Build history of the part. All positions in model axes, mm. A direction names the side the tool comes from. Round coordinates to 2 decimals unless told otherwise and drop trailing zeros. Order: outer loops, then holes, each group sorted by start corner. A loop starts at its lowest first (then second) coordinate and runs counter-clockwise, first axis right, second up. Notation, with made-up numbers: M 83,-32 L 103,-32 A22 ccw 103,-21 Z; hole C -11,17.25 d8. An arc over 180 degrees is marked long. One line per item, written item: value. Start each with the question number.
Item 1: Two-plate mould, pull along Z, no slides. Class faces 4 (the flat face through (15, 86, -42.61)), 5 (the flat face through (25, 69, -62.61)), 6 (the flat face through (162.537, 69, 8)): +Z half, -Z half, draft (parallel to the pull), parting line (faces both ways), or undercut.
Item 2: Band-saw the part on A-A, the plane x = 82.5. Write the cut outline in (y, z).
Item 3: Band-saw the part on B-B, the plane y = 132. Write the cut outline in (x, z), then the cut area to 3 significant figures.
Item 4: Probe L1, parallel to Z at x = 61, y = 136; L2, parallel to Y at x = -86, z = -30.5; L3, parallel to Z at x = 123.5, y = 128. List the from-to ranges inside material, lowest first.
Item 5: Pin check, flat tips, straight feed: pin 1 (5 mm diameter, centred on x = -89.46, z = 7.39, fed in from -Y); pin 2 (1 mm diameter, centred on x = 134.5, y = 97.5, fed in from +Z); pin 3 (6.5 mm diameter, centred on y = 11.5, z = 18.5, fed in from -X); pin 4 (4 mm diameter, centred on x = 108, z = 78, fed in from +Y). Stop position of each tip, or through.
Item 6: Band-saw the part on D-D, the plane y = 113. Write the cut outline in (x, z).
Item 7: Tool access for faces 1 (the flat face through (142.537, 86, 8)), 2 (the flat face through (115.537, 135, 93)), 3 (the flat face through (-60, 20, 7)): list every direction of +Z, -Z, +X, -X, +Y, -Y with a clear straight run to the whole face (end or side of a thin tool).
Item 8: Band-saw the part on C-C, the plane z = -32.5. Write the cut outline in (x, y).
```python
from build123d import *

# Parameters (mm, degrees)
SKETCH_1_W          = 272
SKETCH_1_H          = 140
EXTRUDE_1_DEPTH     = 140
SKETCH_2_W          = 252
SKETCH_2_H          = 100
CUT_EXTRUDE_1_DEPTH = 110
SKETCH_3_W          = 100
SKETCH_3_H          = 13
CUT_EXTRUDE_2_DEPTH = 100
SKETCH_7_R          = 3
CUT_EXTRUDE_3_DEPTH = 211.967749748
SKETCH_8_W          = 12
SKETCH_8_H          = 12
EXTRUDE_2_DEPTH     = 10
SKETCH_9_R          = 14.49
SKETCH_9_R_2        = 4.49
EXTRUDE_1_2_DEPTH   = 12
SKETCH_11_R         = 4.49
CUT_EXTRUDE_5_DEPTH = 298.354040116


with BuildPart() as part:
    # 草圖1 → Extrude 1 (new body)
    with BuildSketch(Plane(origin=(0, 0, 0), x_dir=(1, 0, 0), z_dir=(0, 1, 0))):
        with Locations((26.536585366, -7.390243902)):
            Rectangle(SKETCH_1_W, SKETCH_1_H)
    extrude(amount=EXTRUDE_1_DEPTH)

    # 草圖2 → 除料-伸長1 (cut)
    with BuildSketch(Plane(origin=(0, 140, 0), x_dir=(1, 0, 0), z_dir=(0, 1, 0))):
        with Locations((16.536585366, -7.390243902)):
            Rectangle(SKETCH_2_W, SKETCH_2_H)
    extrude(amount=-CUT_EXTRUDE_1_DEPTH, mode=Mode.SUBTRACT)

    # 草圖3 → 除料-伸長2 (cut)
    with BuildSketch(Plane.ZY.offset(109.463414634)):
        with Locations((7.390243902, 13.5)):
            Rectangle(SKETCH_3_W, SKETCH_3_H)
    extrude(amount=-CUT_EXTRUDE_2_DEPTH, mode=Mode.SUBTRACT)

    # 草圖7 → 除料-伸長3 (cut, through all)
    with BuildSketch(Plane(origin=(0, 30, 0), x_dir=(1, 0, 0), z_dir=(0, 1, 0))):
        with Locations(Location((-89.463414634, -7.390243902, 0), (0, 0, 270))):
            Circle(SKETCH_7_R)
    extrude(amount=-CUT_EXTRUDE_3_DEPTH, mode=Mode.SUBTRACT)

    # 草圖8 → 填料-伸長2 (add)
    with BuildSketch(Plane.XY.offset(77.390243902)):
        with Locations((121.536585366, 126)):
            Rectangle(SKETCH_8_W, SKETCH_8_H)
    extrude(amount=EXTRUDE_2_DEPTH)

    # 草圖9 → Extrude 1 2 (add)
    with BuildSketch(Plane(origin=(127.536585366, 0, 0), x_dir=(0, 0, -1), z_dir=(1, 0, 0))):
        with Locations((-89.390243902, 132)):
            Circle(SKETCH_9_R)
        with Locations((-89.390243902, 132)):
            Circle(SKETCH_9_R_2, mode=Mode.SUBTRACT)
    extrude(amount=-EXTRUDE_1_2_DEPTH)

    # 草圖11 → 除料-伸長5 (cut, through all)
    with BuildSketch(Plane(origin=(127.536585366, 0, 0), x_dir=(0, 0, -1), z_dir=(1, 0, 0))):
        with Locations((-89.390243902, 132)):
            Circle(SKETCH_11_R)
    extrude(amount=-CUT_EXTRUDE_5_DEPTH, mode=Mode.SUBTRACT)


solid = part.part
```
Output:
1. face 4: undercut
1. face 5: -Z half
1. face 6: draft
2. outline: M 0,-62.61 L 140,-62.61 L 140,-42.61 L 30,-42.61 L 30,57.39 L 140,57.39 L 140,77.39 L 0,77.39 Z
3. outline: M -109.46,-62.61 L 162.54,-62.61 L 162.54,77.39 L 127.54,77.39 L 127.54,84.9 L 115.54,84.9 L 115.54,77.39 L -109.46,77.39 L -109.46,57.39 L 142.54,57.39 L 142.54,-42.61 L -109.46,-42.61 Z; M 115.54,93.88 L 127.54,93.88 L 127.54,103.88 L 115.54,103.88 Z
3. area: 13,100 mm²
4. L1: z = -62.61 to -42.61, 57.39 to 77.39
4. L2: y = 0 to 7, 20 to 30
4. L3: z = -62.61 to -42.61, 57.39 to 87.35, 91.43 to 103.32
5. pin 1: passes through
5. pin 2: stops at z = 77.39
5. pin 3: stops at x = -9.46
5. pin 4: stops at y = 140
6. outline: M -109.46,-62.61 L 162.54,-62.61 L 162.54,77.39 L -109.46,77.39 L -109.46,57.39 L 142.54,57.39 L 142.54,-42.61 L -109.46,-42.61 Z
7. face 1: -X, +Y
7. face 2: +Z, -X, +Y, -Y
7. face 3: -X
8. outline: M -109.46,0 L 162.54,0 L 162.54,140 L 142.54,140 L 142.54,30 L -109.46,30 L -109.46,20 L -9.46,20 L -9.46,7 L -109.46,7 Z
